```python
from build123d import *

# Parameters (mm, degrees)
SKETCH1_W           = 60
SKETCH1_H           = 90
BOSS_EXTRUDE1_DEPTH = 15
SKETCH2_R           = 15
BOSS_EXTRUDE2_DEPTH = 30
SKETCH3_R           = 8
BOSS_EXTRUDE5_DEPTH = 15


with BuildPart() as part:
    # Sketch1 → Boss-Extrude1 (new body)
    with BuildSketch(Plane.XY):
        with Locations((-7.135767077, -19.469160134)):
            Rectangle(SKETCH1_W, SKETCH1_H)
    extrude(amount=BOSS_EXTRUDE1_DEPTH)

    # Sketch2 → Boss-Extrude2 (add)
    with BuildSketch(Plane.XY.offset(15)):
        with BuildLine():
            Line((-11.135767077, -49.201297629), (-11.135767077, -52.469160134))
            Line((-11.135767077, -52.469160134), (-3.135767077, -52.469160134))
            Line((-3.135767077, -52.469160134), (-3.135767077, -49.201297629))
            ThreePointArc((-3.135767077, -49.201297629), (-7.135767077, 10.530839866), (-11.135767077, -49.201297629))
        make_face()
        with Locations((-7.135767077, -19.469160134)):
            Circle(SKETCH2_R, mode=Mode.SUBTRACT)
    extrude(amount=BOSS_EXTRUDE2_DEPTH)

    # Sketch3 → Boss-Extrude5 (add)
    with BuildSketch(Plane(origin=(0, 25.530839866, 0), x_dir=(1, 0, 0), z_dir=(0, 1, 0))):
        with BuildLine():
            Line((-7.135767077, 0), (-37.135767077, 0))
            Line((-37.135767077, 0), (-27.151506269, 27.74903454))
            ThreePointArc((-27.151506269, 27.74903454), (-4.217160927, 42.925858918), (16.869139504, 25.271167514))
            Line((16.869139504, 25.271167514), (22.864232923, 0))
            Line((22.864232923, 0), (-7.135767077, 0))
        make_face()
        with Locations((-5.509756001, 19.962209426)):
            Circle(SKETCH3_R, mode=Mode.SUBTRACT)
    extrude(amount=-BOSS_EXTRUDE5_DEPTH)


solid = part.part
```
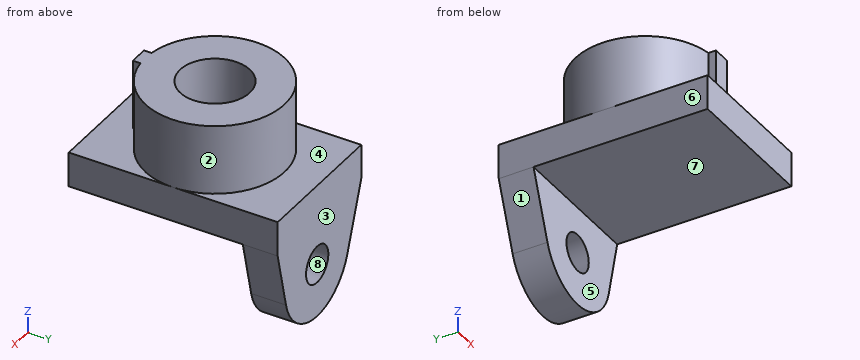
CAD build for the part. Positions are in the model's coordinates, mm. Face numbers are marked on the shaded views. A direction names the side the tool comes from. Coordinates: 2 decimals unless noted, no trailing zeros. Write each loop counter-clockwise with the first axis right and the second up, starting at its lowest first coordinate (ties: lowest second). Pieces come first, ordered by that corner, then holes. Notation, with made-up numbers: (-12.5, 8.5) -> (-1.5, 8.5) arc R17 ccw to (-1.5, 32.5) -> close; hole circle Ø9 at (34, -30). An arc over 180 degrees is marked (long way). Use CSV: the item, a comma, the result in double quotes. Start each with the question number.
Item 1: Band-saw the part on B-B, the plane z = -24. Write the cut outline in (x, y), plus the area to 3 significant figures.
Item 2: Two-plate mould, pull along Z, no slides. Class the marked faces 6, 7 and 8: +Z half, -Z half, draft (parallel to the pull), parting line (faces both ways), or undercut.
Item 3: Tool access for the marked faces 1, 2, 3, 4 and 5: list every direction of +Z, -Z, +X, -X, +Y, -Y with a clear straight run to the whole face (end or side of a thin tool).
Item 4: Band-saw the part on D-D, the plane x = -29.5. Write the cut outline in (y, z).
Item 5: Drop flat-ended pins along their axis: P1, Ø1, axis at y = 9.5, z = -29.5, coming from the -X side; P2, Ø4, axis at y = -24, z = 30.5, coming from the -X side; P3, Ø5, axis at y = 8.5, z = -25, coming from the -X side; P4, Ø3.5, axis at y = -51.5, z = 35.5, coming from the -X side. Give the stop position or say it passes through.
Item 6: Band-saw the part on A-A, the plane z = 20.5. Write the cut outline in (x, y).
Item 7: Band-saw the part on C-C, the plane y = 3. Write the cut outline in (x, z), plus the area to 3 significant figures.
Item 8: Wall check: probe 1 along Z at (x, y) = (-19.5, -10.5); probe 2 along Z at (x, y) = (-17.5, -58.5); probe 3 along Y at (x, z) = (-10.5, -32). Give the ranges that are in metal, low to high.
Response values:
1,outline,"(-28.5, 10.53) -> (-12.42, 10.53) -> (-12.42, 25.53) -> (-28.5, 25.53) -> close; (1.4, 10.53) -> (17.17, 10.53) -> (17.17, 25.53) -> (1.4, 25.53) -> close"
1,area,"478 mm2"
2,face 6,"draft"
2,face 7,"-Z half"
2,face 8,"undercut"
3,face 1,"-Z, -X, +Y, -Y"
3,face 2,"+Z"
3,face 3,"+Z, -Z, +X, -X, +Y"
3,face 4,"+Z, +Y"
3,face 5,"-Z, +X, -X, -Y"
4,outline,"(-64.47, 0) -> (10.53, 0) -> (10.53, -21.22) -> (25.53, -21.22) -> (25.53, 15) -> (0.53, 15) -> (0.53, 45) -> (-39.47, 45) -> (-39.47, 15) -> (-64.47, 15) -> close"
5,P1,"passes through"
5,P2,"stops at x = -37.03"
5,P3,"stops at x = -28.67"
5,P4,"stops at x = -11.14"
6,outline,"(-11.14, -52.47) -> (-3.14, -52.47) -> (-3.14, -49.2) arc R30 ccw (long way) to (-11.14, -49.2) -> close; hole circle Ø30 at (-7.14, -19.47)"
7,outline,"(-37.14, 0) -> (22.86, 0) -> (22.86, 15) -> (12.74, 15) -> (12.74, 45) -> (-27.01, 45) -> (-27.01, 15) -> (-37.14, 15) -> close"
7,area,"2,090 mm2"
8,probe 1,"z = 0 to 45"
8,probe 2,"z = 0 to 15"
8,probe 3,"y = 10.53 to 25.53"
